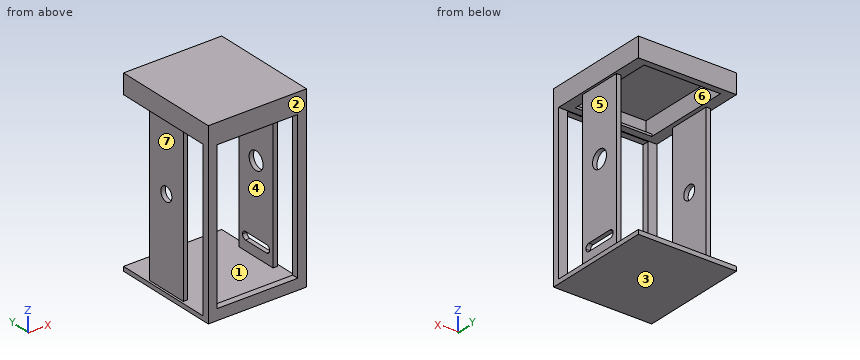
Autodesk Fusion 360 part; units mm, degrees
sketch "Sketch1" plane through (0, 0, 0) normal (0, 0, 1) x (1, 0, 0)
  line L0 (0, 20) -> (45, 20)
  line L1 (45, 20) -> (45, -30)
  line L2 (45, -30) -> (0, -30)
  line L3 (0, -30) -> (0, 20)
  dimension "d1" = 50
  dimension "d2" = 45
extrude "Extrude1" add sketch "Sketch1" along normal blind 2
sketch "Sketch2" plane through (0, 0, 2) normal (0, 0, 1) x (-1, 0, 0)
  line L0 (0, 30) -> (-45, 30)
  line L1 (-45, 30) -> (-45, -20)
  line L2 (-45, -20) -> (0, -20)
  line L3 (0, -20) -> (0, 30)
  line L4 (-1, -6) -> (-3, -6)
  line L5 (-3, -6) -> (-3, 14)
  line L6 (-3, 14) -> (-1, 14)
  line L7 (-1, 14) -> (-1, -6)
  line L8 (-42, -5.8571) -> (-44, -5.8571)
  line L9 (-44, -5.8571) -> (-44, 14.1429)
  line L10 (-44, 14.1429) -> (-42, 14.1429)
  line L11 (-42, 14.1429) -> (-42, -5.8571)
  line L12 (-45, -20) -> (-45, 30)
  line L13 (0, 27) -> (-45, 27)
  line L14 (-45, 27) -> (-45, 30)
  line L15 (-45, 30) -> (0, 30)
  line L16 (0, 30) -> (0, 27)
  dimension "d5" = 20
  dimension "d6" = 2
  dimension "d10" = 2
  dimension "d11" = 39
  dimension "d44" = 1
extrude "Extrude2" add sketch "Sketch2" along normal blind 50 contours L4 L5 L6 L7 | L8 L9 L10 L11
sketch "Sketch3" plane through (42, 0, 0) normal (-1, 0, 0) x (0, -1, 0)
  line L0 (-5.8571, 2) -> (14.1429, 2)
  line L1 (14.1429, 2) -> (14.1429, 52)
  line L2 (14.1429, 52) -> (-5.8571, 52)
  line L3 (-5.8571, 52) -> (-5.8571, 2)
  circle A0 centre (4.1429, 42) radius 4.1125
  dimension "d15" = 8.225
  dimension "d16" = 40
  dimension "d34" = 10
extrude "Extrude3" cut sketch "Sketch3" against normal blind 2 contours A0
sketch "Sketch4" plane through (1, 0, 0) normal (-1, 0, 0) x (0, -1, 0)
  line L0 (-6, 2) -> (14, 2)
  line L1 (14, 2) -> (14, 52)
  line L2 (14, 52) -> (-6, 52)
  line L3 (-6, 52) -> (-6, 2)
  circle A0 centre (4, 42) radius 3.25
  dimension "d19" = 6.5
  dimension "d33" = 10
  dimension "d41" = 10
extrude "Extrude4" cut sketch "Sketch4" against normal blind 2 contours A0
extrude "Extrude5" add sketch "Sketch2" along normal blind 80 contours L0 L1 L3 L12 L13 L14 L15 L16
sketch "Sketch6" plane through (0, -30, 0) normal (0, -1, 0) x (1, 0, 0)
  line L0 (0, 0) -> (45, 0)
  line L1 (45, 0) -> (45, 82)
  line L2 (0, 82) -> (0, 0)
  line L3 (4, 79) -> (41, 79)
  line L4 (41, 79) -> (41, 5)
  line L5 (41, 5) -> (4, 5)
  line L6 (4, 5) -> (4, 79)
  line L7 (45, 82) -> (0, 82)
  dimension "d49" = 74
  dimension "d50" = 5
  dimension "d63" = 37
  dimension "d64" = 4
extrude "Extrude6" cut sketch "Sketch6" against normal blind 3 contours L3 L4 L5 L6
extrude "Extrude9" add 1 faces at (16.3333, -29, 79) along direction (0, 0, -1) blind 1.25
extrude "Extrude10" add 2 faces at (43.3333, -0.8095, 52) (1.6667, -0.6667, 52) along direction (0, 0, 1) blind 26
sketch "Sketch9" plane through (0, -27, 0) normal (0, 1, 0) x (-1, 0, 0)
  line L0 (-45, 2) -> (0, 2)
  line L1 (0, 2) -> (0, 82)
  line L2 (0, 82) -> (-45, 82)
  line L3 (-45, 82) -> (-45, 2)
  line L4 (-45, 82) -> (0, 82)
  line L5 (0, 82) -> (0, 73)
  line L6 (0, 73) -> (-45, 73)
  line L7 (-45, 73) -> (-45, 82)
  line L8 (-41, 5) -> (-41, 77.75)
  line L9 (-41, 77.75) -> (-4, 77.75)
  line L10 (-4, 77.75) -> (-4, 5)
  line L11 (-4, 5) -> (-41, 5)
  dimension "d51" = 9
extrude "Extrude11" add sketch "Sketch9" along normal blind 37 contours L1 L2 L3 L4 L5 L6 L7 L8 L9 L10 | L6 L8 L9 L10
extrude "Extrude12" add 1 faces at (30, 10, 79) along direction (0, 1, 0) blind 5
sketch "Sketch10" plane through (0, 0, 73) normal (0, 0, -1) x (1, 0, 0)
  line L0 (1, -6) -> (1, 14)
  line L1 (1, 14) -> (3, 14)
  line L2 (3, 14) -> (3, -6)
  line L3 (3, -6) -> (1, -6)
  line L4 (42, -5.8571) -> (42, 14.1429)
  line L5 (42, 14.1429) -> (44, 14.1429)
  line L6 (44, 14.1429) -> (44, -5.8571)
  line L7 (44, -5.8571) -> (42, -5.8571)
  line L8 (4, 27) -> (0, 27)
  line L9 (0, 27) -> (0, -15)
  line L10 (0, -15) -> (45, -15)
  line L11 (45, -15) -> (45, 27)
  line L12 (40, -12.6) -> (5, -12.6)
  line L13 (5, -12.6) -> (5, 25)
  line L14 (5, 25) -> (40, 25)
  line L15 (40, 25) -> (40, -12.6)
  line L16 (45, 27) -> (41, 27)
  line L17 (41, 27) -> (4, 27)
  line L18 (40, 25) -> (5, 25)
  line L19 (5, 25) -> (5, 27)
  line L20 (5, 27) -> (40, 27)
  line L21 (40, 27) -> (40, 25)
  dimension "d74" = 2
  dimension "d75" = 37.6
extrude "Extrude13" cut sketch "Sketch10" against normal blind 8 contours L12 L13 L14 L15 L18
extrude "Extrude14" add 1 faces at (16.3333, -29, 77.75) along direction (0, 0, -1) blind 5
extrude "Extrude15" cut sketch "Sketch10" against normal blind 8 contours L14 L17 L18 L19 L20 L21
sketch "Sketch11" plane through (0, -27, 0) normal (0, 1, 0) x (-1, 0, 0)
  line L0 (-4, 72.75) -> (-4, 5)
  line L1 (-4, 5) -> (-41, 5)
  line L2 (-41, 5) -> (-41, 72.75)
  line L3 (-41, 72.75) -> (-4, 72.75)
  line L4 (0, 73) -> (-5, 73)
  line L5 (-5, 73) -> (-5, 81)
  line L6 (-5, 81) -> (-40, 81)
  line L7 (-40, 81) -> (-40, 73)
  line L8 (-40, 73) -> (-45, 73)
  line L9 (-45, 73) -> (-45, 2)
  line L10 (-45, 2) -> (0, 2)
  line L11 (0, 2) -> (0, 73)
  line L12 (-40, 74) -> (-5, 74)
  line L13 (-5, 74) -> (-5, 73)
  line L14 (-5, 73) -> (-40, 73)
  line L15 (-40, 73) -> (-40, 74)
extrude "Extrude16" add sketch "Sketch11" along normal blind 3.5 contours L5 L7 L12 L13 L14 L15
sketch "Sketch12" plane through (44, 0, 0) normal (1, 0, 0) x (0, 1, 0)
  line L0 (5.8571, 73) -> (-14.1429, 73)
  line L1 (-14.1429, 73) -> (-14.1429, 2)
  line L2 (-14.1429, 2) -> (5.8571, 2)
  line L3 (5.8571, 2) -> (5.8571, 73)
  circle A0 centre (-4.1429, 42) radius 4.1125
  line L4 (-12.1429, 10) -> (3.8571, 10)
  line L5 (3.8571, 10) -> (3.8571, 6.5)
  line L6 (3.8571, 6.5) -> (-12.1429, 6.5)
  line L7 (-12.1429, 6.5) -> (-12.1429, 10)
  dimension "d65" = 3.5
  dimension "d66" = 2
  dimension "d67" = 16
extrude "Extrude17" cut sketch "Sketch12" against normal blind 2 contours L4 L5 L6 L7
fillet "Fillet1" radius 1.75 4 edges at (43, 3.8571, 6.5) (43, 3.8571, 10) (43, -12.1429, 10) (43, -12.1429, 6.5)
extrude "Extrude18" add 1 faces at (30, 15, 79) along direction (0, 1, 0) blind 5
sketch "Sketch13" plane through (0, 0, 73) normal (0, 0, -1) x (1, 0, 0)
  line L0 (40, 23.5) -> (40, -12.6)
  line L1 (40, -12.6) -> (5, -12.6)
  line L2 (5, -12.6) -> (5, 23.5)
  line L3 (5, 23.5) -> (40, 23.5)
  line L4 (45, 27) -> (0, 27)
  line L5 (0, 27) -> (0, -20)
  line L6 (0, -20) -> (45, -20)
  line L7 (45, -20) -> (45, 27)
  line L8 (1, -6) -> (1, 14)
  line L9 (1, 14) -> (3, 14)
  line L10 (3, 14) -> (3, -6)
  line L11 (3, -6) -> (1, -6)
  line L12 (42, -5.8571) -> (42, 14.1429)
  line L13 (42, 14.1429) -> (44, 14.1429)
  line L14 (44, 14.1429) -> (44, -5.8571)
  line L15 (44, -5.8571) -> (42, -5.8571)
  line L16 (40, -12.6) -> (5, -12.6)
  line L17 (5, -12.6) -> (5, -17)
  line L18 (5, -17) -> (40, -17)
  line L19 (40, -17) -> (40, -12.6)
extrude "Extrude19" cut sketch "Sketch13" against normal blind 8 contours L1 L16 L17 L18 L19
For this review, take the finished solid that the model builds, in its own axes (mm). Face numbers are marked on the shaded views. A direction names the side the tool comes from. Round coordinates to 2 decimals unless told otherwise and drop trailing zeros. Write each loop counter-clockwise with the first axis right and the second up, starting at its lowest first coordinate (ties: lowest second). Pieces come first, ordered by that corner, then holes. Notation, with made-up numbers: (70.25, -14) - (122.25, -14) arc R20 cw to (122.25, 4) - close; hole circle Ø7 at (-2.5, -0.75). An arc over 180 degrees is marked (long way). Use a Markdown table: item, result.
Q1. We need section D-D (y = -2.5). State how many separate pieces and enclosed holes the cut face has, plus the area to 3 significant figures.
Derived:
| item | result |
|---|---|
| separate pieces | 3 |
| enclosed holes | 0 |
| area | 465 mm2 |
Q2. Clearance check with flat-ended pins moving along their axes: pin 1 (6 mm diameter, centred on y = -5, z = 29, fed in from -X); pin 2 (10 mm diameter, centred on y = 0, z = 43.5, fed in from +X); pin 3 (1.6 mm diameter, centred on x = 42.5, z = 22, fed in from +Y). State where each tip first meets the part, or that it passes through.
Derived:
| item | result |
|---|---|
| pin 1 | stops at x = 1 |
| pin 2 | stops at x = 44 |
| pin 3 | stops at y = 5.86 |
Q3. Machinability: for the marked faces 4, 5, 6 and 7, which of the approach directions +Z, -Z, +X, -X, +Y, -Y give a long, thin tool a straight path to every point of the face, cutting with its end or side? Answer none if there is none.
Derived:
| item | result |
|---|---|
| face 4 | +Y |
| face 5 | +X, +Y |
| face 6 | none |
| face 7 | -X, +Y |
Q4. We need section C-C (x = 14). Give the boundary of the cut face in (y, z).
Derived:
| item | result |
|---|---|
| outline | (-30, 0) - (20, 0) - (20, 2) - (-27, 2) - (-27, 5) - (-30, 5) - close; (-30, 72.75) - (-27, 72.75) - (-27, 73) - (-23.5, 73) - (-23.5, 74) - (-27, 74) - (-27, 81) - (17, 81) - (17, 73) - (20, 73) - (20, 82) - (-30, 82) - close |
Q5. Wall thickness on line 1 along Z through (x, y) = (33.5, -24); line 2 along X through (y, z) = (2.5, 41); line 3 along Z through (x, y) = (32.5, 2): over which ranges is each line inside the solid? List them lowest first.
Derived:
| item | result |
|---|---|
| line 1 | z = 0 to 2, 73 to 74, 81 to 82 |
| line 2 | x = 1 to 3, 42 to 44 |
| line 3 | z = 0 to 2, 81 to 82 |
Q6. The part is to be moulded in two halves that separate along Z. For the marked faces 1, 2 and 3, say which applies: pulls with the +Z half, pulls with the -Z half, needs draft (parallel to the pull), parting line crosses it, or undercut.
Derived:
| item | result |
|---|---|
| face 1 | undercut |
| face 2 | needs draft |
| face 3 | pulls with the -Z half |
Q7. We need section B-B (z = 48.5). Give the boundary of the cut face in (x, y).
Derived:
| item | result |
|---|---|
| outline | (0, -30) - (4, -30) - (4, -27) - (0, -27) - close; (1, -14) - (3, -14) - (3, 6) - (1, 6) - close; (41, -30) - (45, -30) - (45, -27) - (41, -27) - close; (42, -14.14) - (44, -14.14) - (44, 5.86) - (42, 5.86) - close |
Q8. We need section A-A (y = 9.5). Give the boundary of the cut face in (x, z), plus the area to 3 significant figures.
Derived:
| item | result |
|---|---|
| outline | (0, 0) - (45, 0) - (45, 2) - (0, 2) - close; (0, 73) - (5, 73) - (5, 81) - (40, 81) - (40, 73) - (45, 73) - (45, 82) - (0, 82) - close |
| area | 215 mm2 |
